Build history of the part. All positions in model axes, mm. Face numbers are marked on the shaded views. A direction names the side the tool comes from. Round coordinates to 2 decimals unless told otherwise and drop trailing zeros. Order: outer loops, then holes, each group sorted by start corner. A loop starts at its lowest first (then second) coordinate and runs counter-clockwise, first axis right, second up. Notation, with made-up numbers: (75, 62) -> (88, 62) arc R21 ccw to (88, 77) -> close; hole circle Ø8 at (-28.5, 56.25). An arc over 180 degrees is marked (long way). Use a Markdown table: item, result. Add a question column.
Item 1: Pin check, flat tips, straight feed: pin 1 (2 mm diameter, centred on x = -10.5, y = -1.5, fed in from -Z); pin 2 (1.5 mm diameter, centred on y = -0.5, z = -3, fed in from -X). Stop position of each tip, or through.
Item 2: Two-plate mould, pull along X, no slides. Class the marked faces 1, 2 and 3: released by +X, released by -X, zero draft, split by the parting line, or undercut.
Item 3: Slice it at B-B, the plane y = -1.75. Give the cut face in (x, z).
Item 4: Slice it at C-C, the plane x = 0. Give the cut face in (y, z), plus the area to 3 significant figures.
Item 5: Probe L1, parallel to Y at x = -8.75, z = -1.25; L2, parallel to Y at x = 11.25, z = -1.25; L3, parallel to X at y = -1.25, z = -1.5. List the from-to ranges inside material, lowest first.
Item 6: Slice it at D-D, the plane z = -3. Give the cut face in (x, y), plus the area to 3 significant figures.
Item 7: 3-axis set-ups, long thin cutter, end or side, ignore diameter. For the marked faces 4, 5, 6, 7 and 8: which of +Z, -Z, +X, -X, +Y, -Y reach the whole face in a straight line?
Item 8: Slice it at A-A, the plane z = -4.75. Give the cut face in (x, y).
from build123d import *

# Parameters (mm, degrees)
F0_W     = 5
F0_H     = 2
F1_DEPTH = 2.5
F2_W     = 3
F2_H     = 1
F2_W_2   = 2
F3_DEPTH = 25
F5_DEPTH = 25


with BuildPart() as f1:
    # F0 (on Front) → F1 (new body, symmetric)
    with BuildSketch(Plane.XZ):
        with BuildLine():
            ThreePointArc((5.25, 0), (0, -5.25), (-5.25, 0))
            Line((-5.25, 0), (-7.25, 0))
            ThreePointArc((-7.25, 0), (-5.126524, -5.126524), (0, -7.25))
            ThreePointArc((0, -7.25), (5.126524, -5.126524), (7.25, 0))
            Line((7.25, 0), (5.25, 0))
        make_face()
        with BuildLine():
            ThreePointArc((0, -7.25), (-5.126524, -5.126524), (-7.25, 0))
            Line((-7.25, 0), (-7.25, -2))
            Line((-7.25, -2), (-7.25, -7.25))
            Line((-7.25, -7.25), (0, -7.25))
        make_face()
        with Locations((-9.75, -1)):
            Rectangle(F0_W, F0_H)
        with BuildLine():
            Line((7.25, -2), (7.25, 0))
            ThreePointArc((7.25, 0), (5.126524, -5.126524), (0, -7.25))
            Line((0, -7.25), (7.25, -7.25))
            Line((7.25, -7.25), (7.25, -2))
        make_face()
        with Locations((9.75, -1)):
            Rectangle(F0_W, F0_H)
    extrude(amount=F1_DEPTH, both=True)

    # F2 (on Top) → F3 (cut)
    with BuildSketch(Plane.XY):
        with Locations((-10.75, 0)):
            Rectangle(F2_W, F2_H)
        with Locations((-8.25, 1)):
            Rectangle(F2_W_2, F2_H)
        with Locations((-8.25, 0)):
            Rectangle(F2_W_2, F2_H)
        with Locations((-8.25, -1)):
            Rectangle(F2_W_2, F2_H)
        with Locations((10.75, 0)):
            Rectangle(F2_W, F2_H)
        with Locations((8.25, 1)):
            Rectangle(F2_W_2, F2_H)
        with Locations((8.25, 0)):
            Rectangle(F2_W_2, F2_H)
        with Locations((8.25, -1)):
            Rectangle(F2_W_2, F2_H)
    extrude(amount=-F3_DEPTH, mode=Mode.SUBTRACT)

    # F4 (on face) → F5 (cut)
    with BuildSketch(Plane.YZ.offset(7.25)):
        Polygon((2.5, -7.25), (2.5, -5.910254), (-2.5, -7.25), align=None)
    extrude(amount=-F5_DEPTH, mode=Mode.SUBTRACT)


solid = f1.part
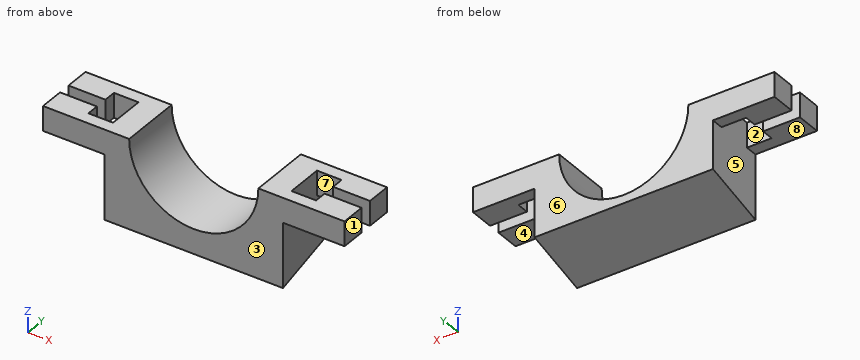
Check sheet entries:
| question | item | result |
|---|---|---|
| 1 | pin 1 | z = -2 |
| 1 | pin 2 | x = -7.25 |
| 2 | face 1 | released by +X |
| 2 | face 2 | undercut |
| 2 | face 3 | zero draft |
| 3 | outline | (-12.25, -2) -> (-7.25, -2) -> (-7.25, -7.05) -> (7.25, -7.05) -> (7.25, -2) -> (12.25, -2) -> (12.25, 0) -> (5.25, 0) arc R5.25 cw to (-5.25, 0) -> (-12.25, 0) -> close |
| 4 | outline | (-2.5, -7.25) -> (2.5, -5.91) -> (2.5, -5.25) -> (-2.5, -5.25) -> close |
| 4 | area | 6.65 mm2 |
| 5 | L1 | -2.5 to -1.5, 1.5 to 2.5 |
| 5 | L2 | -2.5 to -0.5, 0.5 to 2.5 |
| 5 | L3 | -12.25 to -9.25, -7.25 to -5.03, 5.03 to 7.25, 9.25 to 12.25 |
| 6 | outline | (-7.25, -2.5) -> (-4.31, -2.5) -> (-4.31, 2.5) -> (-7.25, 2.5) -> close; (4.31, -2.5) -> (7.25, -2.5) -> (7.25, 2.5) -> (4.31, 2.5) -> close |
| 6 | area | 29.4 mm2 |
| 7 | face 4 | -Z, +X, +Y, -Y |
| 7 | face 5 | -Z |
| 7 | face 6 | +Z, -Z, +X, -X, +Y |
| 7 | face 7 | +Z, -Z |
| 7 | face 8 | -Z, -X, +Y, -Y |
| 8 | outline | (-7.25, -2.5) -> (-2.24, -2.5) -> (-2.24, 2.5) -> (-7.25, 2.5) -> close; (2.24, -2.5) -> (7.25, -2.5) -> (7.25, 2.5) -> (2.24, 2.5) -> close |
